Check sheet for the drawn part. Datum: minimum x, y, z corner. Units: mm. A direction names the side the tool comes from. Coordinates: 2 decimals unless noted, no trailing zeros. Order: outer loops, then holes, each group sorted by start corner. A loop starts at its lowest first (then second) coordinate and runs counter-clockwise, first axis right, second up. Notation, with made-up numbers: (-36.5, -23) - (-32.5, -23) arc R33 cw to (-32.5, 9) - close; hole circle Ø5 at (-26.5, 64). An arc over 180 degrees is marked (long way). Return JSON: item names as keys, results as strings. Group by question number.
Item 1: Section check C-C on z = 3. Enter the section's corners in (x, y).
Item 2: Section check A-A on x = 27. Enter the section's corners in (y, z).
Item 3: Gauge pin test, flat ends, axial feed: pin 1 (1.5 mm diameter, centred on x = 31.5, y = 6, fed in from -Z); pin 2 (3 mm diameter, centred on x = 21, y = 10, fed in from -Z). Record the tip position at first contact, or that the pin passes through.
Item 4: Section check B-B on y = 8. Enter the section's corners in (x, z).
Item 5: Tool access check on the marked faces 4, 5 and 6. Record the directions out of +Z, -Z, +X, -X, +Y, -Y that give a thin tool (end or side, any length) a straight path to the whole face; none if there is none.
Item 6: Draft check along Y on the marked faces 1, 2 and 3. Enter one of: pulls with the +Y half, pulls with the -Y half, needs draft (parallel to the pull), parting line crosses it, or undercut.
Item 7: Scan lines: probe 1 along Y at (x, z) = (39, 8); probe 2 along X at (y, z) = (14.5, 13.25); probe 3 along X at (y, z) = (26, 7.75). Record each from-to range of solid material in increasing order.
Item 8: Section check D-D on x = 4. Enter the section's corners in (y, z).
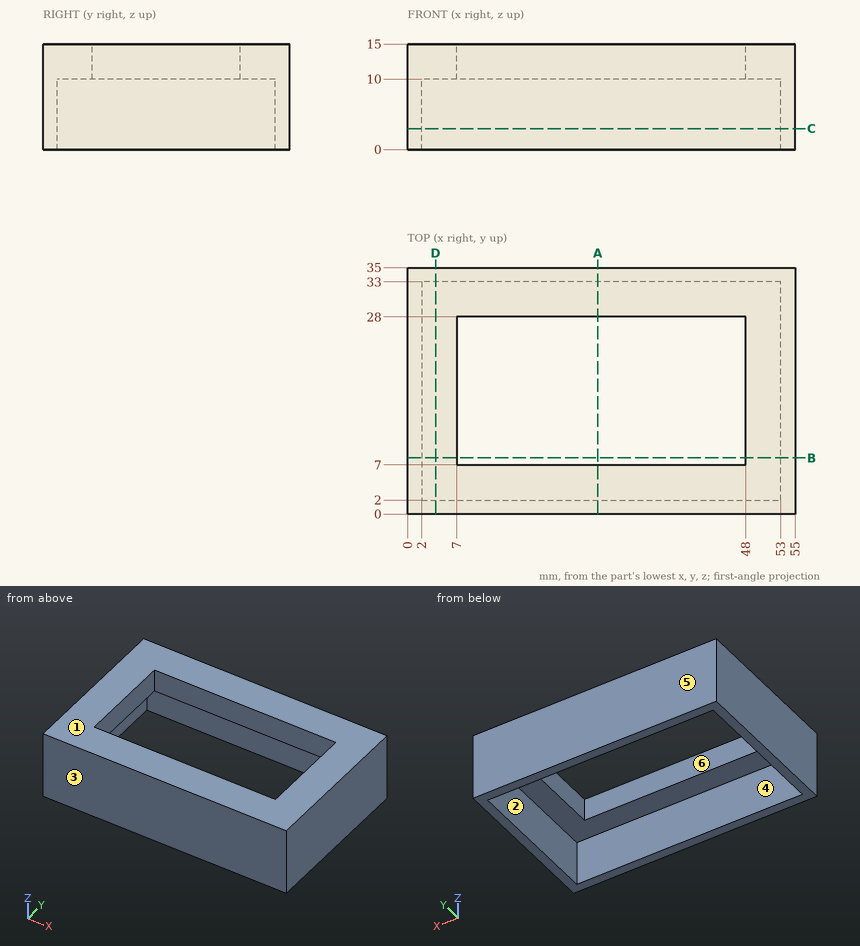
Computed:
{
 "1": {"outline": "(0, 0) - (55, 0) - (55, 35) - (0, 35) - close; hole (2, 2) - (53, 2) - (53, 33) - (2, 33) - close"},
 "2": {"outline": "(0, 0) - (2, 0) - (2, 10) - (7, 10) - (7, 15) - (0, 15) - close; (28, 10) - (33, 10) - (33, 0) - (35, 0) - (35, 15) - (28, 15) - close"},
 "3": {"pin 1": "stops at z = 10", "pin 2": "passes through"},
 "4": {"outline": "(0, 0) - (2, 0) - (2, 10) - (7, 10) - (7, 15) - (0, 15) - close; (48, 10) - (53, 10) - (53, 0) - (55, 0) - (55, 15) - (48, 15) - close"},
 "5": {"face 4": "-Z", "face 5": "+Z, -Z, +X, -X, +Y", "face 6": "+Z, -Z"},
 "6": {"face 1": "needs draft", "face 2": "undercut", "face 3": "pulls with the -Y half"},
 "7": {"probe 1": "y = 0 to 2, 33 to 35", "probe 2": "x = 0 to 7, 48 to 55", "probe 3": "x = 0 to 2, 53 to 55"},
 "8": {"outline": "(0, 0) - (2, 0) - (2, 10) - (33, 10) - (33, 0) - (35, 0) - (35, 15) - (0, 15) - close"}
}
